Check sheet for the modelled part. Datum: model origin and axes. Units: mm. Face numbers are marked on the shaded views. A direction names the side the tool comes from. Give positions to 0.01 mm unless a question says otherwise; leave off trailing zeros. Order: outer loops, then holes, each group sorted by start corner. A loop starts at its lowest first (then second) coordinate and runs counter-clockwise, first axis right, second up. Notation, with made-up numbers: (12, 41) -> (23, 41) arc R20 cw to (23, 71) -> close; hole circle Ø1 at (56, 40.5). An arc over 180 degrees is marked (long way). Answer in a Markdown table with one row per item. Add a question column.
(1) Release check for a two-part mould opening along Y. For the marked faces 3, 4 and 5 record: released by +Y, released by -Y, zero draft, split by the parting line, or undercut.
(2) Go/stop test with flat-tipped pins: pin 1 (13 mm diameter, centred on y = -57, z = -26, fed in from -X); pin 2 (3.5 mm diameter, centred on y = -21.56, z = -23.8, fed in from +X); pin 3 (2 mm diameter, centred on x = 1.5, y = -32, fed in from -Z). Record where each tip stops, or that it passes through.
(3) Cross-section at D-D (y = -31.5). Record the cut outline in (x, z), then the cut area to 3 significant figures.
(4) Set-up check for the marked faces 1 and 2: record each of +Z, -Z, +X, -X, +Y, -Y from which the full face is reachable in a straight line by a thin tool's end or side.
(5) Thickness scan on L1, parallel to Z at x = 4.05, y = -41.5; L2, parallel to Z at x = 3.9, y = -47.5; L3, parallel to X at y = -62, z = -4. Record the ranges inside material, lowest first. Write a range as [from, to].
(6) Cross-section at A-A (y = -43.5). Record the cut outline in (x, z), then the cut area to 3 significant figures.
(7) Cross-section at C-C (x = 1.85). Record the cut outline in (y, z), then the cut area to 3 significant figures.
(8) Cross-section at B-B (z = -5). Record the cut outline in (x, y), then the cut area to 3 significant figures.
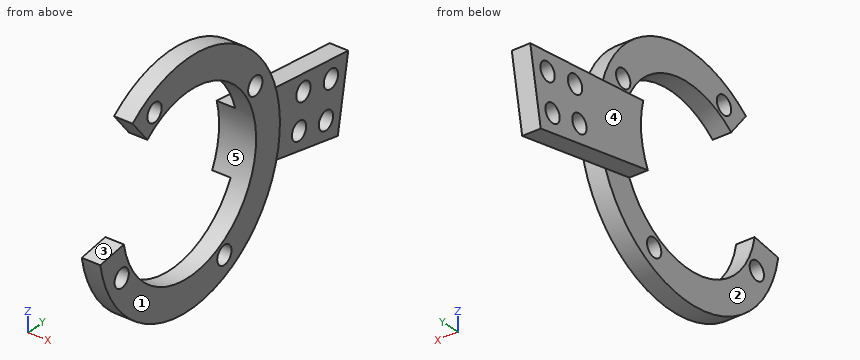
Autodesk Inventor part; units mm, degrees
ref_plane "YZ Plane" through (0, 0, 0) normal (1, 0, 0) x (0, 1, 0)
ref_plane "XZ Plane" through (0, 0, 0) normal (0, 1, 0) x (-1, 0, 0)
ref_plane "XY Plane" through (0, 0, 0) normal (0, 0, 1) x (1, 0, 0)
sketch "Эскиз1" plane through (0, 0, 0) normal (1, 0, 0) x (0, 1, 0)
  circle A0 centre (-54.1058, -16.5076) radius 16
  circle A1 centre (-54.1058, -16.5076) radius 14
  circle A2 centre (-54.1058, -16.5076) radius 19
  line L0 (-54.1058, -16.5076) -> (-62.8101, 0.3813)
  line L1 (-54.1058, -16.5076) -> (-45.4015, -33.3965)
  line L2 (-54.1058, -16.5076) -> (-70.9947, -25.2119)
  line L3 (-54.1058, -16.5076) -> (-37.6871, -6.9458)
  line L4 (-67.8834, -18.9928) -> (-72.8305, -19.73)
  line L5 (-62.9482, -5.6535) -> (-66.048, -1.7298)
  line L6 (-40.6156, -12.7639) -> (-16.8789, -15.5395)
  line L7 (-16.8789, -15.5395) -> (-19.0698, -27.3017)
  line L8 (-19.0698, -27.3017) -> (-41.5699, -22.7407)
  line L9 (-28.383, -14.1943) -> (-30.5675, -24.971)
  line L10 (-28.383, -14.1943) -> (-19.0698, -27.3017)
  line L11 (-30.5675, -24.971) -> (-16.8789, -15.5395)
  line L12 (-23.9604, -20.4186) -> (-22.9207, -14.833)
  line L13 (-22.9207, -14.833) -> (-29.4202, -19.3112)
  line L14 (-22.9207, -14.833) -> (-17.9743, -21.4206)
  line L15 (-23.9604, -20.4186) -> (-24.9531, -26.1091)
  line L16 (-17.9743, -21.4206) -> (-24.9429, -26.0503)
  line L17 (-29.4202, -19.3112) -> (-24.9429, -26.0503)
  circle A3 centre (-61.4358, -2.2854) radius 1.5
  circle A4 centre (-68.328, -23.8376) radius 1.5
  circle A5 centre (-46.7758, -30.7298) radius 1.5
  circle A6 centre (-40.2796, -8.4556) radius 1.5
  circle A7 centre (-26.2831, -17.1497) radius 1.5
  circle A8 centre (-20.5111, -18.0421) radius 1.5
  circle A9 centre (-21.5572, -23.8009) radius 1.5
  circle A10 centre (-27.201, -22.6514) radius 1.5
  point P0 (-6.6177, -23.1834)
  point P1 (-76.739, -12.454)
  point P2 (39.1344, -10.1827)
  point P3 (-35.3653, -13.3778)
  point P4 (-36.5442, -23.7594)
  dimension "d0" = 32
  dimension "d2" = 28
  dimension "d3" = 38
  dimension "d7" = 3
  dimension "d8" = 3
  dimension "d9" = 3
  dimension "d10" = 3
  dimension "d11" = 3
  dimension "d12" = 3
  dimension "d13" = 3
  dimension "d15" = 3
extrude "Выдавливание1" add sketch "Эскиз1" along normal blind 6 contours A0 L8 A1 L6 | A0 L6 A2 L8 | L6 A1 L3 A6 A0 | A0 A6 L3 A2 L6 | L8 A2 L1 A5 A0 | A0 A5 L1 A1 L8 | L3 A1 L0 A3 A0 A6 | L3 A6 A0 A3 L0 A2 | A5 A0 A4 L2 A1 L1 | A2 L2 A4 A0 A5 L1 | A1 L5 A0 A3 L0 | L0 A3 A0 L5 A2 | A2 L4 A0 A4 L2 | L2 A4 A0 L4 A1
extrude "Выдавливание2" add sketch "Эскиз1" along normal blind 3 contours L6 L9 L8 A2 | L10 A7 L13 L9 | L6 L13 A7 L10 | L11 A10 L17 L15 L8 | L9 L17 A10 L11 | L14 A8 L11 L12 | L12 L10 A7 L13 | L6 L11 A8 L14 | L13 A7 L10 L11 A10 L17 | L15 L16 A9 L10 L8 | L7 L14 A8 L11 | L11 A8 L14 L16 A9 L10 | L15 L17 A10 L11 | L10 A9 L16 L15 | L10 A9 L16 L7
extrude "Выдавливание3" cut sketch "Эскиз1" along normal blind 3 contours L6 A1 L3 A6 A0 | A0 A6 L3 A2 L6 | L8 A2 L1 A5 A0 | A0 A5 L1 A1 L8 | L3 A1 L0 A3 A0 A6 | L3 A6 A0 A3 L0 A2 | A5 A0 A4 L2 A1 L1 | A2 L2 A4 A0 A5 L1 | A1 L5 A0 A3 L0 | L0 A3 A0 L5 A2 | A2 L4 A0 A4 L2 | L2 A4 A0 L4 A1
sketch "Эскиз3" plane through (3, 0, 0) normal (-1, 0, 0) x (0, 0, 1)
  line L0 (-32.3349, -33.8419) -> (-22.1169, -29.7797)
  line L1 (-26.451, -18.878) -> (-17.9696, -40.2117)
  line L2 (-26.8452, -44.8668) -> (-37.4977, -23.4738)
  line L3 (-34.7862, -28.919) -> (-27.4833, -31.9131)
  line L4 (-27.4833, -31.9131) -> (-24.288, -24.4799)
  line L5 (-29.5408, -26.736) -> (-24.2332, -24.4564)
  line L6 (-37.4977, -23.4738) -> (-26.451, -18.878)
  line L7 (-31.9743, -21.1759) -> (-24.288, -24.4799)
  line L8 (-34.7862, -28.919) -> (-31.9743, -21.1759)
  line L9 (-22.1169, -29.7797) -> (-37.4977, -23.4738)
  line L10 (-32.3349, -33.8419) -> (-26.451, -18.878)
  line L11 (-29.5408, -26.736) -> (-34.7862, -28.919)
  line L12 (-16.3356, -54.116) -> (-33.3178, -45.5953)
  line L13 (-16.3356, -54.116) -> (-6.9524, -37.5946)
  line L14 (-20.5901, -67.4538) -> (-22.1809, -72.1945)
  line L15 (-16.3356, -54.116) -> (-25.7187, -70.6374)
  line L16 (-16.3356, -54.116) -> (0.1858, -63.4991)
  circle A0 centre (-16.3356, -54.116) radius 14
  circle A1 centre (-16.3356, -54.116) radius 16
  circle A2 centre (-16.3356, -54.116) radius 19
  line L17 (-6.7225, -64.2939) -> (-3.4007, -68.0332)
  circle A3 centre (-24.2372, -68.0287) radius 1.5
  circle A4 centre (-2.4228, -62.0176) radius 1.5
  circle A5 centre (-8.434, -40.2032) radius 1.5
  circle A6 centre (-30.6364, -46.9407) radius 1.5
  circle A7 centre (-31.0082, -30.4679) radius 1.5
  circle A8 centre (-33.4164, -25.147) radius 1.5
  circle A9 centre (-28.0225, -22.8746) radius 1.5
  circle A10 centre (-25.8996, -28.2288) radius 1.5
  point P0 (0, 0)
  point P1 (-7.3565, -75.2836)
  point P2 (-62.9166, -3.4682)
  point P3 (41.7851, -43.7086)
  point P4 (-32.7147, -46.9037)
  point P5 (-33.8935, -57.2853)
  dimension "d22" = 32
  dimension "d23" = 28
  dimension "d24" = 38
  dimension "d25" = 3
  dimension "d26" = 3
  dimension "d27" = 3
  dimension "d28" = 3
  dimension "d29" = 3
  dimension "d30" = 3
  dimension "d31" = 3
  dimension "d32" = 3
properties part number "motor_mound"
Answer below:
| question | item | result |
|---|---|---|
| 1 | face 3 | released by -Y |
| 1 | face 4 | zero draft |
| 1 | face 5 | undercut |
| 2 | pin 1 | stops at x = 3 |
| 2 | pin 2 | stops at x = 3 |
| 2 | pin 3 | stops at z = -24.88 |
| 3 | outline | (0, -24.78) -> (3, -24.78) -> (3, -13.83) -> (0, -13.83) -> close |
| 3 | area | 32.9 mm² |
| 4 | face 1 | +Z, -Z, +X, +Y, -Y |
| 4 | face 2 | -Z, -X, -Y |
| 5 | L1 | z = [-30.72, -22.6], [-10.42, -9.33], [-7.58, -2.29] |
| 5 | L2 | z = [-34.32, -32.04], [-29.42, -28.85], [-4.16, 1.31] |
| 5 | L3 | x = [3, 6] |
| 6 | outline | (3, -32.27) -> (6, -32.27) -> (6, -25.65) -> (3, -25.65) -> close; (3, -7.37) -> (6, -7.37) -> (6, -0.74) -> (3, -0.74) -> close |
| 6 | area | 39.8 mm² |
| 7 | outline | (-41.57, -22.74) -> (-19.07, -27.3) -> (-16.88, -15.54) -> (-40.62, -12.76) arc R14 cw to start; hole circle Ø3 at (-27.2, -22.65); hole circle Ø3 at (-26.28, -17.15); hole circle Ø3 at (-21.56, -23.8); hole circle Ø3 at (-20.51, -18.04) |
| 7 | area | 223 mm² |
| 8 | outline | (3, -63.46) -> (6, -63.46) -> (6, -62.08) -> (3, -62.08) -> close; (3, -46.13) -> (6, -46.13) -> (6, -38.99) -> (3, -38.99) -> close |
| 8 | area | 25.6 mm² |
